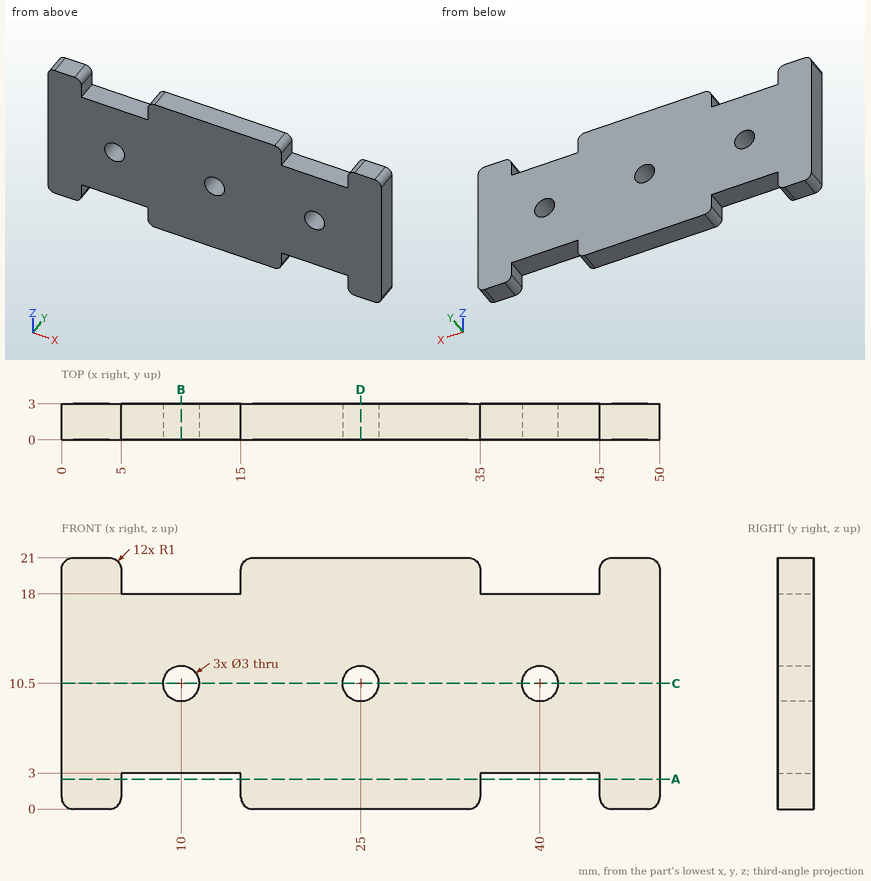
Geometry check sheet. Reference: drawing and pictorial views, mm from the part's lowest x, y, z. Give positions to 0.01 mm unless a question says otherwise; leave off trailing zeros. Loops run counter-clockwise (first coordinate to the right, second up) from the corner with the lowest first, then second, coordinate; pieces in that order, holes last. Notation, with made-up numbers: (72, 14) - (131, 14) arc R9 ccw to (131, 20) - close; hole circle Ø4 at (71, 42.25). An arc over 180 degrees is marked (long way). One line per question, with ' | ' between items. Start each with the question number.
1. Cross-section at A-A, the plane z = 2.5. Enter the section's corners in (x, y), plus the area to 3 significant figures.
2. Cross-section at D-D, the plane x = 25. Enter the section's corners in (y, z).
3. Material ranges on line 1 along X through (y, z) = (1.7, 10.5); line 2 along X through (y, z) = (2.4, 18.75); line 3 along Z through (x, y) = (40, 1.4), recorded low to high. Write a range as [from, to].
4. Cross-section at C-C, the plane z = 10.5. Enter the section's corners in (x, y), plus the area to 3 significant figures.
5. Gauge pin test, flat ends, axial feed: pin 1 Ø1.8 at (x, z) = (25, 10.5) entering from -Y; pin 2 Ø0.9 at (x, y) = (10, 1) entering from +Z. Record the tip position at first contact, or that the pin passes through.
6. Cross-section at B-B, the plane x = 10. Enter the section's corners in (y, z).
Check result:
1) outline: (0, 0) - (5, 0) - (5, 3) - (0, 3) - close; (15, 0) - (35, 0) - (35, 3) - (15, 3) - close; (45, 0) - (50, 0) - (50, 3) - (45, 3) - close | area: 90.0 mm2
2) outline: (0, 0) - (3, 0) - (3, 9) - (0, 9) - close; (0, 12) - (3, 12) - (3, 21) - (0, 21) - close
3) line 1: x = [0, 8.5], [11.5, 23.5], [26.5, 38.5], [41.5, 50] | line 2: x = [0, 5], [15, 35], [45, 50] | line 3: z = [3, 9], [12, 18]
4) outline: (0, 0) - (8.5, 0) - (8.5, 3) - (0, 3) - close; (11.5, 0) - (23.5, 0) - (23.5, 3) - (11.5, 3) - close; (26.5, 0) - (38.5, 0) - (38.5, 3) - (26.5, 3) - close; (41.5, 0) - (50, 0) - (50, 3) - (41.5, 3) - close | area: 123 mm2
5) pin 1: passes through | pin 2: stops at z = 18
6) outline: (0, 3) - (3, 3) - (3, 9) - (0, 9) - close; (0, 12) - (3, 12) - (3, 18) - (0, 18) - close
